Work out the finished part from the listing and answer in its coordinate system (mm). Face numbers are marked on the shaded views. A direction names the side the tool comes from. Coordinates: 2 decimals unless noted, no trailing zeros. Write each loop counter-clockwise with the first axis right and the second up, starting at its lowest first coordinate (ties: lowest second). Pieces come first, ordered by that corner, then holes. Notation, with made-up numbers: M -29.5,43 L 29.5,43 A21 cw 29.5,65 Z; hole C 74,-24.75 d2. An arc over 180 degrees is marked long. Answer as CSV lines item,"result". Start each with the question number.
(1) Find the intervals of material crossed by L1, parallel to X at y = -1.4, z = -0.6; L2, parallel to X at y = -0.2, z = -0.9; L3, parallel to Z at x = 0.75, y = -2.5, in increasing order. Write a range as [from, to].
(2) The mould has two halves that part along Z. Classify the marked faces 1, 2 and 3: released by +Z, released by -Z, zero draft, split by the parting line, or undercut.
(3) A cutting plane is placed at B-B on y = -2.3. Give the vertices of the cut face in (x, z), then the cut area to 3 significant figures.
(4) A cutting plane is placed at A-A on y = -0.4. Give the vertices of the cut face in (x, z).
(5) A flat-ended cylindrical pin translates along its axis: P1, Ø2, axis at x = 0, y = -1.5, coming from the +Z side. Find the tip coordinate at first contact, or state that the pin passes through.
(6) For the marked faces 4, 5 and 6, determine the directions among +Z, -Z, +X, -X, +Y, -Y from which every point of the face is accessible in a straight line to the end or side of a thin tool.
Autodesk Inventor part; units mm, degrees
ref_plane "YZ Plane" through (0, 0, 0) normal (1, 0, 0) x (0, 1, 0)
ref_plane "XZ Plane" through (0, 0, 0) normal (0, 1, 0) x (-1, 0, 0)
ref_plane "XY Plane" through (0, 0, 0) normal (0, 0, 1) x (1, 0, 0)
sketch "Szkic2" plane through (0, 0, 0) normal (1, 0, 0) x (0, 1, 0)
  line L0 (0, -2.9) -> (0, 2.9)
  line L1 (-1.5, -1.5) -> (-1.5, 1.5)
  line L2 (-1.5, -1.5) -> (0, -2.9)
  line L3 (-1.5, 1.5) -> (0, 2.9)
  line L4 (0, 0) -> (-4, 0)
  line L5 (-4, 0) -> (-4, -1.5)
  line L6 (-4, -1.5) -> (-1.5, -1.5)
  dimension "d0" = 5.8
  dimension "d2" = 3
  dimension "d3" = 1.5
  dimension "d4" = 4
  dimension "d5" = 1.5
revolve "Obrót1" add sketch "Szkic2" angle 360 about axis through (0, 0, 0) along (0, -1, 0) contours L2 L1 L4 L0 | L6 L5 L4 L1
sketch "Szkic3" plane through (0, 0, 0) normal (0, 1, 0) x (1, 0, 0)
  line L0 (-1.1673, -0.633) -> (-1.1318, 0.6945)
  line L1 (-1.1318, 0.6945) -> (0.0355, 1.3274)
  line L2 (0.0355, 1.3274) -> (1.1673, 0.633)
  line L3 (1.1673, 0.633) -> (1.1318, -0.6945)
  line L4 (1.1318, -0.6945) -> (-0.0355, -1.3274)
  line L5 (-0.0355, -1.3274) -> (-1.1673, -0.633)
  point P0 (0, 0)
  point P1 (0, 0)
  dimension "d7" = 2.3
extrude "Wyciągnięcie proste1" cut sketch "Szkic3" against normal blind 2
fillet "Zaokrąglenie1" radius 0.5 6 edges at (-1.1496, -2, -0.0308) (-0.6014, -2, 0.9802) (-0.5482, -2, -1.011) (0.6014, -2, -0.9802) (0.5482, -2, 1.011) (1.1496, -2, 0.0308)
fillet "Zaokrąglenie2" radius 0.5 1 edges at (0, -1.5, 1.5)
fillet "Zaokrąglenie3" radius 0.1 1 edges at (0, 0, 2.9)
thread "Gwint1"
chamfer "Faza1" distance 0.5 angle 45 1 edges at (0, -4, 1.5)
properties part number "Screw M3 4mm flat head"
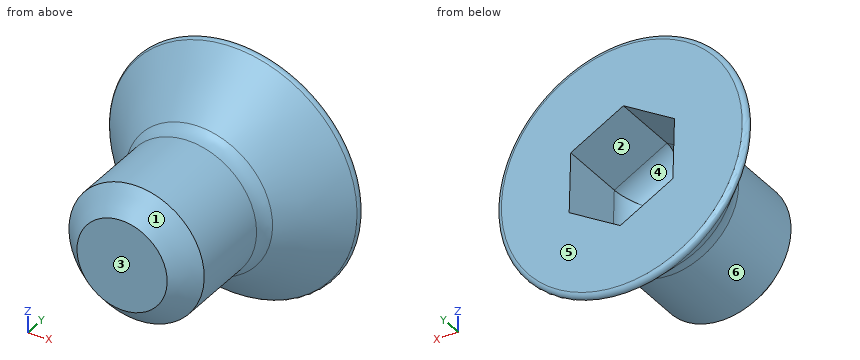
Here are the results:
1,L1,"x = [-1.48, -1.13], [1.17, 1.48]"
1,L2,"x = [-2.56, -0.75], [0.73, 2.56]"
1,L3,"z = [-1.3, 1.3]"
2,face 1,"split by the parting line"
2,face 2,"undercut"
2,face 3,"zero draft"
3,outline,"C 0,0 d3"
3,area,"7.07 mm^2"
4,outline,"C 0,0 d5.05; hole M -1.17,0.63 L -1.13,-0.69 L 0.04,-1.33 L 1.17,-0.63 L 1.13,0.69 L -0.04,1.33 Z"
5,P1,"stops at z = 2.43"
6,face 4,"+Y"
6,face 5,"+Z, -Z, +X, -X, +Y"
6,face 6,"-Y"
